The figure shows three views and two pictorial views of one solid part (mm, origin at its lowest corner). Answer the questions. Coordinates: 2 decimals unless noted, no trailing zeros. Loops run counter-clockwise (first coordinate to the right, second up) from the corner with the lowest first, then second, coordinate; pieces in that order, holes last. Notation, with made-up numbers: M 20.25,-32 L 71.25,-32 A32 ccw 71.25,-1 Z; hole C 9,82 d5. An arc over 180 degrees is marked long. Answer as a JSON object with one key per item and string values. Group by question number.
1. Given pin 1 (3 mm diameter, centred on x = 27.9, y = 15.9, fed in from -Z); pin 2 (5 mm diameter, centred on x = 24.5, y = 4.5, fed in from -Z); pin 3 (9.5 mm diameter, centred on x = 8.5, y = 16.5, fed in from -Z); pin 4 (2 mm diameter, centred on x = 22, z = 2, fed in from +Y), each flat-ended and moving along its own axis, determine where each tip first touches the part or whether it passes through.
2. Determine the mould class of the marked faces 1, 2 and 3 for opening direction Y: released by +Y, released by -Y, zero draft, split by the parting line, or undercut.
3. Straight lines are drawn through the part: L1, parallel to Y at x = 15.9, z = 10.5; L2, parallel to Z at x = 5, y = 24; L3, parallel to X at y = 16, z = 3.75. For each, find the intervals that lie inside material, in ascending order.
4. A cutting plane is placed at D-D on z = 6.75. Give the vertices of the cut face in (x, y).
5. A cutting plane is placed at C-C on z = 11.5. Give the vertices of the cut face in (x, y).
6. A cutting plane is placed at A-A on y = 15.9. Give the vertices of the cut face in (x, z), and give its area (3 significant figures).
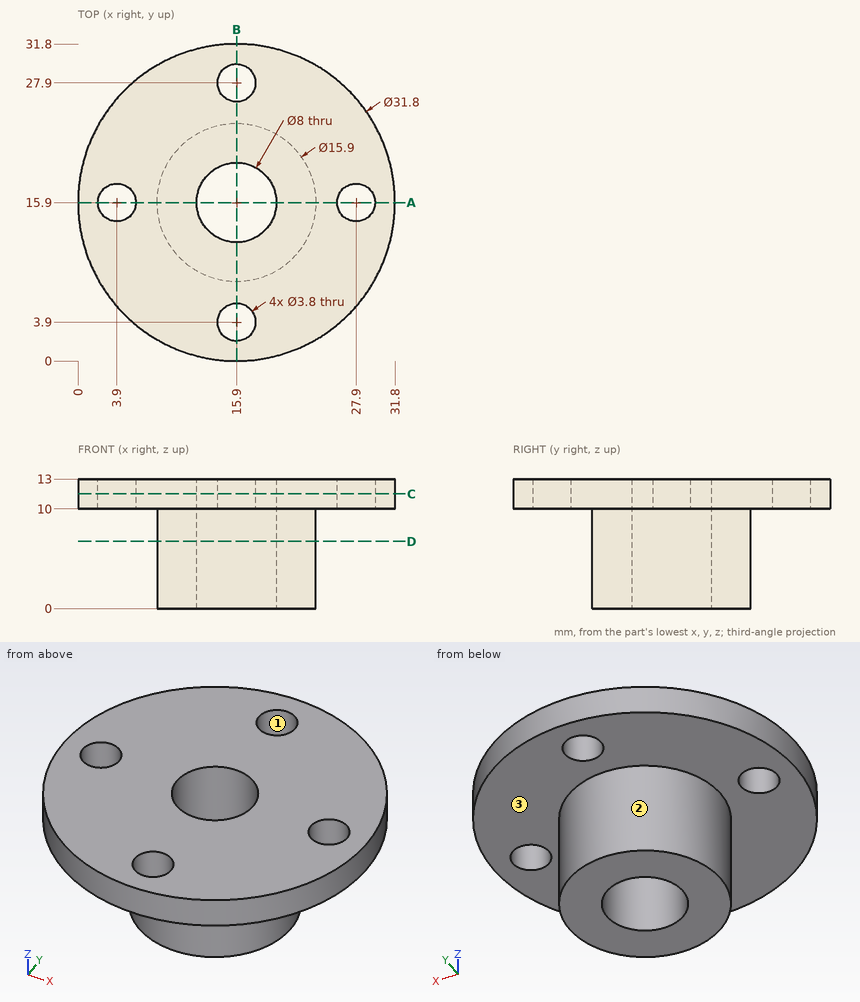
From the geometry:
{
 "1": {"pin 1": "passes through", "pin 2": "stops at z = 10", "pin 3": "stops at z = 0", "pin 4": "stops at y = 22"},
 "2": {"face 1": "undercut", "face 2": "split by the parting line", "face 3": "zero draft"},
 "3": {"L1": "y = 0 to 2, 5.8 to 11.9, 19.9 to 26, 29.8 to 31.8", "L2": "z = 10 to 13", "L3": "x = 7.95 to 11.9, 19.9 to 23.85"},
 "4": {"outline": "C 15.9,15.9 d15.9; hole C 15.9,15.9 d8"},
 "5": {"outline": "C 15.9,15.9 d31.8; hole C 3.9,15.9 d3.8; hole C 15.9,15.9 d8; hole C 15.9,3.9 d3.8; hole C 15.9,27.9 d3.8; hole C 27.9,15.9 d3.8"},
 "6": {"outline": "M 0,10 L 2,10 L 2,13 L 0,13 Z; M 5.8,10 L 7.95,10 L 7.95,0 L 11.9,0 L 11.9,13 L 5.8,13 Z; M 19.9,0 L 23.85,0 L 23.85,10 L 26,10 L 26,13 L 19.9,13 Z; M 29.8,10 L 31.8,10 L 31.8,13 L 29.8,13 Z", "area": "128 mm²"}
}
